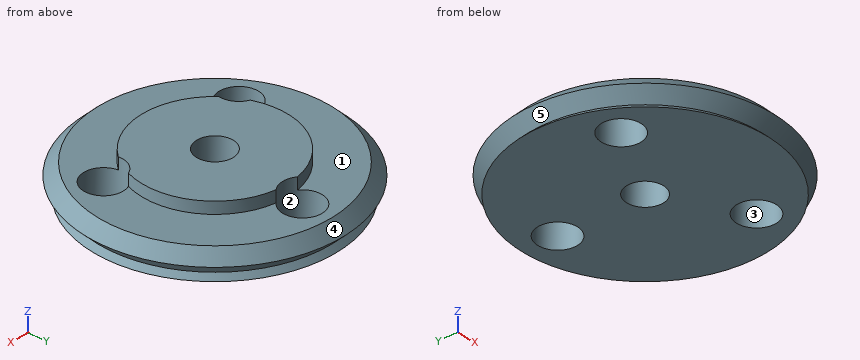
```python
from build123d import *

# Parameters (mm, degrees)
CYLINDER002_R     = 20
CYLINDER002_DEPTH = 20
CYLINDER001_R     = 1.35
CYLINDER001_DEPTH = 10
ARRAY001_COUNT    = 3
CYLINDER_R        = 4.1
CYLINDER_DEPTH    = 2.25
SKETCH002_W       = 5
SKETCH002_H       = 4.7
ARRAY_Z_COUNT     = 6
ARRAY_Z_PITCH     = 1.6


with BuildPart() as upperdomain:
    # Cylinder002 → Cylinder002 (new body)
    with BuildSketch(Plane.XY.offset(1.25)):
        Circle(CYLINDER002_R)
    extrude(amount=CYLINDER002_DEPTH)


with BuildPart() as obj1:
    # Cylinder001 → Cylinder001 (new body)
    with BuildSketch(Plane(origin=(0, 6, -4), x_dir=(1, 0, 0), z_dir=(0, 0, 1))):
        Circle(CYLINDER001_R)
    extrude(amount=CYLINDER001_DEPTH)

    # Array001: obj1 ×3 about axis
    array001_axis = Axis((0, 0, 0), (0, 0, 1))


with BuildPart() as obj1_1:
    add(obj1.part)
    for i in range(1, ARRAY001_COUNT):
        add(obj1.part.rotate(array001_axis, i * 360 / ARRAY001_COUNT))


with BuildPart() as lensfit:
    # Cylinder → Cylinder (new body)
    with BuildSketch(Plane.XY.offset(-1)):
        Circle(CYLINDER_R)
    extrude(amount=CYLINDER_DEPTH)


with BuildPart() as obj2:
    # Sketch002 → Revolution002 (revolve)
    with BuildSketch(Plane.XZ):
        with Locations((7.5, 0.85)):
            Rectangle(SKETCH002_W, SKETCH002_H)
    revolve(axis=Axis((0, 0, 0), (0, 0, 1)))


with BuildPart() as innergroovetool:
    # Sketch001 → Revolution001 (revolve)
    with BuildSketch(Plane.XZ):
        Polygon((4, 3.2), (4, 1.6), (8, 1.6), (8.8, 2.4), (8, 3.2), align=None)
    revolve(axis=Axis((0, 0, 0), (0, 0, 1)))

    # Array Z: InnerGrooveTool ×6


with BuildPart() as innergroovetool_1:
    add(innergroovetool.part)
    with Locations(*[(0, 0, -i * ARRAY_Z_PITCH) for i in range(1, ARRAY_Z_COUNT)]):
        add(innergroovetool.part)

    # Common: intersect obj2
    add(obj2.part, mode=Mode.INTERSECT)


with BuildPart() as lid:
    # Sketch → Revolution (revolve)
    with BuildSketch(Plane.XZ):
        Polygon((1.25, 4), (1.25, -1.5), (8, -1.5), (8, 3.2), (5, 3.2), (5, 4), align=None)
    revolve(axis=Axis((0, 0, 0), (0, 0, 1)))

    # Fusion001: union InnerGrooveTool
    add(innergroovetool_1.part)

    # Cut: cut LensFit
    add(lensfit.part, mode=Mode.SUBTRACT)

    # Cut001: cut obj1
    add(obj1_1.part, mode=Mode.SUBTRACT)

    # Common001: intersect UpperDomain
    add(upperdomain.part, mode=Mode.INTERSECT)


solid = lid.part
```
The listing builds one solid part. Answer for the finished solid, in the listing's coordinates (mm). Face numbers are marked on the shaded views. A direction names the side the tool comes from. Coordinates: 2 decimals unless noted, no trailing zeros. Loops run counter-clockwise (first coordinate to the right, second up) from the corner with the lowest first, then second, coordinate; pieces in that order, holes last. Notation, with made-up numbers: (53.25, 86.5) - (70.25, 86.5) arc R18 ccw to (70.25, 119.5) - close; hole circle Ø2 at (77, 59). An arc over 180 degrees is marked (long way). Use a Markdown table: item, result. Add a question column.
1) The mould has two halves that part along Z. Classify the marked faces 3, 4 and 5: released by +Z, released by -Z, zero draft, split by the parting line, or undercut.
2) For the marked faces 1 and 2, determine the directions among +Z, -Z, +X, -X, +Y, -Y from which every point of the face is accessible in a straight line to the end or side of a thin tool.
3) The part is cut by section A-A, the plane y = 0. Give the vertices of the cut face in (x, z).
4) The part is cut by section B-B, the plane x = 0. Give the vertices of the cut face in (y, z), and give its area (3 significant figures).
5) Find the intervals of material crossed by line 1 (Y direction, x = 0, z = 3.35); line 2 (Z direction, x = -5.5, y = 1.25); line 3 (Y direction, x = 0.5, z = 1.4), in increasing order.
6) The part is cut by section C-C, the plane z = 1.9. Give the vertices of the cut face in (x, y), and give its area (3 significant figures).
Here are the results:
| question | item | result |
|---|---|---|
| 1 | face 3 | zero draft |
| 1 | face 4 | released by +Z |
| 1 | face 5 | undercut |
| 2 | face 1 | +Z |
| 2 | face 2 | +Z, -Z |
| 3 | outline | (-8.8, 2.4) - (-8, 1.6) - (-8.35, 1.25) - (-1.25, 1.25) - (-1.25, 4) - (-5, 4) - (-5, 3.2) - (-8, 3.2) - close; (1.25, 1.25) - (8.35, 1.25) - (8, 1.6) - (8.8, 2.4) - (8, 3.2) - (5, 3.2) - (5, 4) - (1.25, 4) - close |
| 4 | outline | (-8.8, 2.4) - (-8, 1.6) - (-8.35, 1.25) - (-1.25, 1.25) - (-1.25, 4) - (-5, 4) - (-5, 3.2) - (-8, 3.2) - close; (1.25, 1.25) - (4.65, 1.25) - (4.65, 4) - (1.25, 4) - close; (7.35, 1.25) - (8.35, 1.25) - (8, 1.6) - (8.8, 2.4) - (8, 3.2) - (7.35, 3.2) - close |
| 4 | area | 28.2 mm^2 |
| 5 | line 1 | y = -5 to -1.25, 1.25 to 4.65 |
| 5 | line 2 | z = 1.25 to 3.2 |
| 5 | line 3 | y = -8.18 to -1.15, 1.15 to 4.75, 7.25 to 8.18 |
| 6 | outline | circle Ø16.6 at (0, 0); hole circle Ø2.7 at (-5.2, -3); hole circle Ø2.7 at (0, 6); hole circle Ø2.5 at (0, 0); hole circle Ø2.7 at (5.2, -3) |
| 6 | area | 194 mm^2 |
